```python
from build123d import *

# Parameters (mm, degrees)
SKETCH001_R      = 8
SKETCH001_R_2    = 2.6
EXTRUDE001_DEPTH = 15
SKETCH_W         = 70
SKETCH_H         = 40
SKETCH_R         = 6
EXTRUDE_DEPTH    = 7
SKETCH002_W      = 70
SKETCH002_H      = 10
EXTRUDE002_DEPTH = 3


with BuildPart() as extrude001:
    # Sketch001 → Extrude001 (new body)
    with BuildSketch(Plane.XY):
        with Locations((-25, -12)):
            Circle(SKETCH001_R)
        with Locations((-25, -12)):
            Circle(SKETCH001_R_2, mode=Mode.SUBTRACT)
        with Locations((25, -12)):
            Circle(SKETCH001_R)
        with Locations((25, -12)):
            Circle(SKETCH001_R_2, mode=Mode.SUBTRACT)
    extrude(amount=EXTRUDE001_DEPTH)


with BuildPart() as extrude_body:
    # Sketch → Extrude (new body)
    with BuildSketch(Plane.XY):
        Rectangle(SKETCH_W, SKETCH_H)
        with Locations((-25, -12)):
            Circle(SKETCH_R, mode=Mode.SUBTRACT)
        with Locations((25, -12)):
            Circle(SKETCH_R, mode=Mode.SUBTRACT)
    extrude(amount=EXTRUDE_DEPTH)


with BuildPart() as fusion:
    # Sketch002 → Extrude002 (new body)
    with BuildSketch(Plane.XY):
        with Locations((0, 15)):
            Rectangle(SKETCH002_W, SKETCH002_H)
    extrude(amount=EXTRUDE002_DEPTH)


with BuildPart() as fusion_1:
    # Extrude002 placement: moved
    add(fusion.part.moved(Location((0, 0, 7))))

    # Fusion: union Extrude001, Extrude body
    add(extrude001.part)
    add(extrude_body.part)


solid = fusion_1.part
```
Input: part model. Units: mm. Frame: model coordinates. A direction names the side the tool comes from. Give positions to 0.01 mm unless a question says otherwise; leave off trailing zeros. Loops run counter-clockwise (first coordinate to the right, second up) from the corner with the lowest first, then second, coordinate; pieces in that order, holes last. Notation, with made-up numbers: (5.25, 30) -> (49.25, 30) arc R13 cw to (49.25, 49) -> close; hole circle Ø11 at (73.5, -6). An arc over 180 degrees is marked (long way). Use a Markdown table: item, result.
Q1. Section query A-A, the plane z = 7.75. Return the cut outline in (x, y).
Entries:
| item | result |
|---|---|
| outline | (-35, 10) -> (35, 10) -> (35, 20) -> (-35, 20) -> close; circle Ø16 at (-25, -12); circle Ø16 at (25, -12); hole circle Ø5.2 at (-25, -12); hole circle Ø5.2 at (25, -12) |
Q2. Access query for faces 5 (the cylindrical face through (18.651, -16.868, 10.944)), 6 (the flat face through (-27, -10, 15)), 7 (the flat face through (0, 10, 8)), 8 (the flat face through (0, 15, 10)), 9 (the flat face through (35, 0, 4)). Directions: +Z, -Z, +X, -X, +Y, -Y. A direction counts if a zero-diameter tool reaches every point of the face in a straight line with its end or side. Return the directions, or none.
Entries:
| item | result |
|---|---|
| face 5 | +Z |
| face 6 | +Z, +X, -X, +Y, -Y |
| face 7 | +Z, +X, -X |
| face 8 | +Z, +X, -X, +Y |
| face 9 | +Z, -Z, +X, +Y, -Y |
Q3. Section query D-D, the plane x = -10. Return the cut outline in (y, z), plus the area to 3 significant figures.
Entries:
| item | result |
|---|---|
| outline | (-20, 0) -> (20, 0) -> (20, 10) -> (10, 10) -> (10, 7) -> (-20, 7) -> close |
| area | 310 mm² |
Q4. Pull-direction query (X, two-part tool) for faces 1 (the flat face through (0, 0, 0)), 2 (the cylindrical face through (-31.349, -16.868, 10.944)), 3 (the flat face through (-35, 0, 4)), 4 (the cylindrical face through (-23.8, -14.307, 7.395)); classes: pulls with the +X half, pulls with the -X half, needs draft (parallel to the pull), parting line crosses it, or undercut.
Entries:
| item | result |
|---|---|
| face 1 | needs draft |
| face 2 | undercut |
| face 3 | pulls with the -X half |
| face 4 | undercut |
Q5. Section query C-C, the plane z = 1.5. Return the cut outline in (x, y), plus the area to 3 significant figures.
Entries:
| item | result |
|---|---|
| outline | (-35, -20) -> (35, -20) -> (35, 20) -> (-35, 20) -> close; hole circle Ø5.2 at (-25, -12); hole circle Ø5.2 at (25, -12) |
| area | 2,760 mm² |
Q6. Section query B-B, the plane y = -12. Return the cut outline in (x, z), plus the area to 3 significant figures.
Entries:
| item | result |
|---|---|
| outline | (-35, 0) -> (-27.6, 0) -> (-27.6, 15) -> (-33, 15) -> (-33, 7) -> (-35, 7) -> close; (-22.4, 0) -> (22.4, 0) -> (22.4, 15) -> (17, 15) -> (17, 7) -> (-17, 7) -> (-17, 15) -> (-22.4, 15) -> close; (27.6, 0) -> (35, 0) -> (35, 7) -> (33, 7) -> (33, 15) -> (27.6, 15) -> close |
| area | 590 mm² |
Q7. First-contact query: P1, Ø2, axis at x = -15, y = -15, coming from the +Z side; P2, Ø12, axis at x = 16.5, y = 5, coming from the +Z side; P3, Ø10, axis at x = 7.5, y = 16, coming from the -Z side; P4, Ø3, axis at x = -25, y = -12, coming from the +Z side. Flat tips, straight axial feed; report the tip coordinate or a pass-through.
Entries:
| item | result |
|---|---|
| P1 | stops at z = 7 |
| P2 | stops at z = 10 |
| P3 | stops at z = 0 |
| P4 | passes through |
Q8. Ray query, probe 1 along Y at (x, z) = (25, 8.75); probe 2 along Y at (x, z) = (-25, 6.75); probe 3 along Z at (x, y) = (11.5, 13.5). Return the intervals inside material, ascending. Write a range as from..to.
Entries:
| item | result |
|---|---|
| probe 1 | y = -20..-14.6, -9.4..-4, 10..20 |
| probe 2 | y = -20..-14.6, -9.4..20 |
| probe 3 | z = 0..10 |
